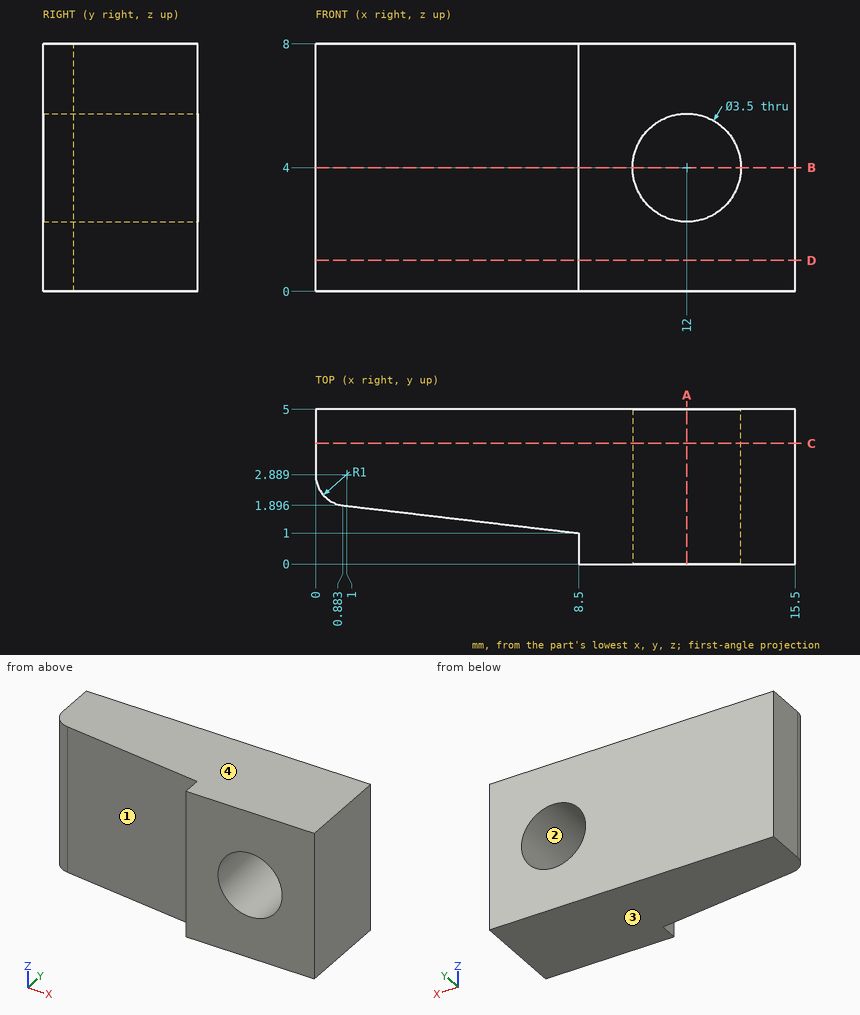
Study the drawing (mm; zero at the part's minimum x, y, z) and answer. Give positions to 0.01 mm unless a question says otherwise; leave off trailing zeros. Write each loop counter-clockwise with the first axis right and the second up, starting at its lowest first coordinate (ties: lowest second). Pieces come first, ordered by that corner, then holes.
Item 1: Find the intervals of material crossed by line 1 along Z through (x, y) = (12, 3.9); line 2 along X through (y, z) = (3.15, 3.75); line 3 along Z through (x, y) = (11.25, 3.5), in increasing order.
Item 2: Section C-C, the plane y = 3.9 is taken. Write down the section's boundary in (x, z).
Item 3: Section D-D, the plane z = 1 is taken. Write down the section's boundary in (x, y).
Item 4: Flat-ended cylindrical pins translate along their axes: P1, Ø3, axis at x = 12, z = 4, coming from the +Y side; P2, Ø0.8, axis at y = 0.5, z = 3.5, coming from the -X side. Find the tip coordinate at first contact, or state that the pin passes through.
Item 5: Section B-B, the plane z = 4 is taken. Write down the section's boundary in (x, y).
Item 6: Determine the mould class of the marked faces 1, 2, 3 and 4 for opening direction Z: released by +Z, released by -Z, zero draft, split by the parting line, or undercut.
Item 7: Section A-A, the plane x = 12 is taken. Write down the section's boundary in (y, z), plus the area to 3 significant figures.
Completed:
1. line 1: z = 0 to 2.25, 5.75 to 8
1. line 2: x = 0 to 10.27, 13.73 to 15.5
1. line 3: z = 0 to 2.42, 5.58 to 8
2. outline: (0, 0) - (15.5, 0) - (15.5, 8) - (0, 8) - close; hole circle Ø3.5 at (12, 4)
3. outline: (0, 2.89) arc R1 ccw to (0.88, 1.9) - (8.5, 1) - (8.5, 0) - (15.5, 0) - (15.5, 5) - (0, 5) - close
4. P1: passes through
4. P2: stops at x = 8.5
5. outline: (0, 2.89) arc R1 ccw to (0.88, 1.9) - (8.5, 1) - (8.5, 0) - (10.25, 0) - (10.25, 5) - (0, 5) - close; (13.75, 0) - (15.5, 0) - (15.5, 5) - (13.75, 5) - close
6. face 1: zero draft
6. face 2: undercut
6. face 3: released by -Z
6. face 4: released by +Z
7. outline: (0, 0) - (5, 0) - (5, 2.25) - (0, 2.25) - close; (0, 5.75) - (5, 5.75) - (5, 8) - (0, 8) - close
7. area: 22.5 mm2
